CAD build for the part. Positions are in the model's coordinates, mm. Coordinates: 2 decimals unless noted, no trailing zeros. Write each loop counter-clockwise with the first axis right and the second up, starting at its lowest first coordinate (ties: lowest second). Pieces come first, ordered by that corner, then holes. Notation, with made-up numbers: (20.25, -7.5) - (72.25, -7.5) arc R10 cw to (72.25, 11.5) - close; hole circle Ø4 at (-28.75, 85.25). An arc over 180 degrees is marked (long way). Answer in a Markdown table with one row per item. Add a question column.
Q1. Band-saw the part on D-D (x = 11). List the corners of the cut face in (y, z).
Q2. Band-saw the part on B-B (y = 3). List the corners of the cut face in (x, z).
Q3. Two-plate mould, pull along X, no slides. Class faces 1 (the flat face through (0, 12, 4)), 2 (the cylindrical face through (9.4, 13.87, 1.77)), 3 (the flat face through (21, 23.8, 4)): +X half, -X half, draft (parallel to the pull), parting line (faces both ways), or undercut.
Q4. Band-saw the part on A-A (x = 22.5). List the corners of the cut face in (y, z).
Q5. Pin check, flat tip, straight feed: pin 1 (1.6 mm diameter, centred on x = 22.5, y = 3, fed in from +Z). Stop position of the tip, or through.
Q6. Band-saw the part on C-C (z = 5.5). List the corners of the cut face in (x, y).
Q7. Drill centre lines: line 1 along Y through (x, z) = (3, 2.5); line 2 along X through (y, z) = (2.75, 1.25); line 3 along Y through (x, z) = (11, 2.7). Where is each one in solid material? Low to high. Write a range as from..to.
```python
from build123d import *

# Parameters (mm, degrees)
SKETCH030_W     = 42
SKETCH030_H     = 23.8
PAD019_DEPTH    = 8
SKETCH032_R     = 1.6
SKETCH032_R_2   = 1.3
POCKET010_DEPTH = 8.001
CHAMFER002_SIZE = 4.5


with BuildPart() as part:
    # Sketch030 → Pad019 (new body)
    with BuildSketch(Plane.XY):
        with Locations((21, 11.9)):
            Rectangle(SKETCH030_W, SKETCH030_H)
    extrude(amount=PAD019_DEPTH)

    # Sketch032 (on Face6 of Pad019) → Pocket010 (cut, through all)
    with BuildSketch(Plane.XY.offset(8)):
        with Locations((11, 13.8)):
            Circle(SKETCH032_R)
        with Locations((31, 13.8)):
            Circle(SKETCH032_R)
        with Locations((3, 3)):
            Circle(SKETCH032_R_2)
        with Locations((22.5, 3)):
            Circle(SKETCH032_R_2)
    extrude(amount=-POCKET010_DEPTH, mode=Mode.SUBTRACT)

    # Chamfer002
    chamfer002_edges = [part.edges().sort_by_distance(p)[0] for p in [
        (9.4, 13.8, 8),
        (29.4, 13.8, 8),
    ]]
    chamfer(chamfer002_edges, length=CHAMFER002_SIZE)


solid = part.part
```
Checked values:
| question | item | result |
|---|---|---|
| 1 | outline | (0, 0) - (12.2, 0) - (12.2, 3.5) - (7.7, 8) - (0, 8) - close; (15.4, 0) - (23.8, 0) - (23.8, 8) - (19.9, 8) - (15.4, 3.5) - close |
| 2 | outline | (0, 0) - (1.7, 0) - (1.7, 8) - (0, 8) - close; (4.3, 0) - (21.2, 0) - (21.2, 8) - (4.3, 8) - close; (23.8, 0) - (42, 0) - (42, 8) - (23.8, 8) - close |
| 3 | face 1 | -X half |
| 3 | face 2 | undercut |
| 3 | face 3 | draft |
| 4 | outline | (0, 0) - (1.7, 0) - (1.7, 8) - (0, 8) - close; (4.3, 0) - (23.8, 0) - (23.8, 8) - (4.3, 8) - close |
| 5 | pin 1 | passes through |
| 6 | outline | (0, 0) - (42, 0) - (42, 23.8) - (0, 23.8) - close; hole circle Ø2.6 at (3, 3); hole circle Ø7.2 at (11, 13.8); hole circle Ø2.6 at (22.5, 3); hole circle Ø7.2 at (31, 13.8) |
| 7 | line 1 | y = 0..1.7, 4.3..23.8 |
| 7 | line 2 | x = 0..1.72, 4.28..21.22, 23.78..42 |
| 7 | line 3 | y = 0..12.2, 15.4..23.8 |
